Can you work these out from the model? Positions are in its coordinate system, mm. A direction names the side the tool comes from. Give positions to 0.01 mm unless a question says otherwise; leave off trailing zeros. Write each loop counter-clockwise with the first axis right and the second up, starting at its lowest first coordinate (ties: lowest second). Pieces come first, ordered by that corner, then holes.
from build123d import *

# Parameters (mm, degrees)
SKETCH2_W           = 60
SKETCH2_H           = 60
BOSS_EXTRUDE1_DEPTH = 10
SKETCH3_R           = 2
CUT_EXTRUDE1_DEPTH  = 10
SKETCH4_R           = 6.35
CUT_EXTRUDE2_DEPTH  = 3.2
SKETCH5_R           = 2.7
CUT_EXTRUDE3_DEPTH  = 7
SKETCH6_R           = 0.5
CUT_EXTRUDE4_DEPTH  = 3


with BuildPart() as part:
    # Sketch2 → Boss-Extrude1 (new body)
    with BuildSketch(Plane(origin=(0, 0, 0), x_dir=(1, 0, 0), z_dir=(0, 1, 0))):
        Rectangle(SKETCH2_W, SKETCH2_H)
    extrude(amount=BOSS_EXTRUDE1_DEPTH)

    # Sketch3 → Cut-Extrude1 (cut)
    with BuildSketch(Plane(origin=(0, 10, 0), x_dir=(1, 0, 0), z_dir=(0, 1, 0))):
        with Locations((-26, 26)):
            Circle(SKETCH3_R)
        with Locations((-26, -26)):
            Circle(SKETCH3_R)
        with Locations((0, -26)):
            Circle(SKETCH3_R)
        with Locations((26, -26)):
            Circle(SKETCH3_R)
        with Locations((26, 26)):
            Circle(SKETCH3_R)
        with Locations((0, 26)):
            Circle(SKETCH3_R)
    extrude(amount=-CUT_EXTRUDE1_DEPTH, mode=Mode.SUBTRACT)

    # Sketch4 → Cut-Extrude2 (cut)
    with BuildSketch(Plane.XZ):
        Circle(SKETCH4_R)
    extrude(amount=-CUT_EXTRUDE2_DEPTH, mode=Mode.SUBTRACT)

    # Sketch5 → Cut-Extrude3 (cut)
    with BuildSketch(Plane(origin=(0, 10, 0), x_dir=(1, 0, 0), z_dir=(0, 1, 0))):
        with Locations((12.5, 0)):
            Circle(SKETCH5_R)
        with Locations((-12.5, 0)):
            Circle(SKETCH5_R)
    extrude(amount=-CUT_EXTRUDE3_DEPTH, mode=Mode.SUBTRACT)

    # Sketch6 → Cut-Extrude4 (cut)
    with BuildSketch(Plane.XZ):
        with Locations((12.5, 0)):
            Circle(SKETCH6_R)
        with Locations((-12.5, 0)):
            Circle(SKETCH6_R)
    extrude(amount=-CUT_EXTRUDE4_DEPTH, mode=Mode.SUBTRACT)


solid = part.part
(1) Imagine slicing it at D-D, the plane x = 26. Write out the boundary of the cut face in (y, z), plus the area to 3 significant figures.
Returned:
outline: (0, -30) - (10, -30) - (10, -28) - (0, -28) - close; (0, -24) - (10, -24) - (10, 24) - (0, 24) - close; (0, 28) - (10, 28) - (10, 30) - (0, 30) - close
area: 520 mm2
(2) If we mould it in two halves opening along Z, with no side actions, what happens to faces 1 (the face through (0, 10, 0)), 2 (the face through (-26, 5, -24)), 3 (the face through (0, 5, 30))? For each: +Z half, -Z half, draft (parallel to the pull), parting line (faces both ways), or undercut.
Returned:
face 1: draft
face 2: undercut
face 3: +Z half
(3) Will these pins go through, and if not, where does the flat tip stop? P1, Ø16.5, axis at x = 0, z = 0, coming from the -Y side; P2, Ø3.5, axis at x = 0, z = 26, coming from the +Y side; P3, Ø2.5, axis at x = -13.5, z = -1, coming from the +Y side.
Returned:
P1: stops at y = 0
P2: passes through
P3: stops at y = 3
(4) Imagine slicing it at C-C, the plane x = 0. Write out the boundary of the cut face in (y, z).
Returned:
outline: (0, -30) - (10, -30) - (10, -28) - (0, -28) - close; (0, -24) - (10, -24) - (10, 24) - (0, 24) - (0, 6.35) - (3.2, 6.35) - (3.2, -6.35) - (0, -6.35) - close; (0, 28) - (10, 28) - (10, 30) - (0, 30) - close
(5) For faces 4 (the face through (-30, 5, 0)), 5 (the face through (12, 3, 1)), 6 (the face through (0, 3.2, 0)), which set-ups out of +Z, -Z, +X, -X, +Y, -Y let a thin tool reach every point of the face, with its end or its side?
Returned:
face 4: +Z, -Z, -X, +Y, -Y
face 5: +Y
face 6: -Y
(6) If I drill on L1, parallel to X at y = 8.25, z = 26; L2, parallel to X at y = 6, z = -24.5; L3, parallel to Z at x = 12.5, y = 1.4, over which ranges is the centre line in solid material (lowest first)?
Returned:
L1: x = -30 to -28, -24 to -2, 2 to 24, 28 to 30
L2: x = -30 to -27.32, -24.68 to -1.32, 1.32 to 24.68, 27.32 to 30
L3: z = -30 to -0.5, 0.5 to 30
(7) Imagine slicing it at A-A, the plane z = -26. Write out the boundary of the cut face in (x, y), plus the area to 3 significant figures.
Returned:
outline: (-30, 0) - (-28, 0) - (-28, 10) - (-30, 10) - close; (-24, 0) - (-2, 0) - (-2, 10) - (-24, 10) - close; (2, 0) - (24, 0) - (24, 10) - (2, 10) - close; (28, 0) - (30, 0) - (30, 10) - (28, 10) - close
area: 480 mm2
(8) Imagine slicing it at B-B, the plane y = 7. Give the number of separate pieces and of enclosed holes in the cut face, plus the area to 3 significant figures.
Returned:
separate pieces: 1
enclosed holes: 8
area: 3,480 mm2
